from build123d import *

# Parameters (mm, degrees)
SKETCH1_R           = 2.1
BOSS_EXTRUDE1_DEPTH = 3
SKETCH2_W           = 4
SKETCH2_H           = 24
BOSS_EXTRUDE2_DEPTH = 15
SKETCH5_R           = 2.1
CUT_EXTRUDE3_DEPTH  = 65
FILLET2_R           = 2
FILLET3_R           = 3
SKETCH6_W           = 30
SKETCH6_H           = 5
BOSS_EXTRUDE3_DEPTH = 8
FILLET5_R           = 2
SKETCH9_R           = 2.1
CUT_EXTRUDE8_DEPTH  = 34


with BuildPart() as part:
    # Sketch1 → Boss-Extrude1 (new body)
    with BuildSketch(Plane(origin=(0, 0, 0), x_dir=(1, 0, 0), z_dir=(0, 1, 0))):
        Polygon((-20.9, -20.9), (20.9, -20.9), (20.9, -12), (28, -12), (28, 12), (20.9, 12), (20.9, 20.9), (-20.9, 20.9), (-20.9, 12), (-28, 12), (-28, -12), (-20.9, -12), align=None)
        with Locations(Location((-16, 16, 0), (0, 0, 270))):
            Circle(SKETCH1_R, mode=Mode.SUBTRACT)
        with Locations(Location((16, 16, 0), (0, 0, 270))):
            Circle(SKETCH1_R, mode=Mode.SUBTRACT)
        with Locations(Location((16, -16, 0), (0, 0, 270))):
            Circle(SKETCH1_R, mode=Mode.SUBTRACT)
        with Locations(Location((-16, -16, 0), (0, 0, 270))):
            Circle(SKETCH1_R, mode=Mode.SUBTRACT)
    extrude(amount=BOSS_EXTRUDE1_DEPTH)

    # Sketch2 → Boss-Extrude2 (add)
    with BuildSketch(Plane(origin=(0, 3, 0), x_dir=(1, 0, 0), z_dir=(0, 1, 0))):
        with Locations((-26, 0)):
            Rectangle(SKETCH2_W, SKETCH2_H)
        with Locations((26, 0)):
            Rectangle(SKETCH2_W, SKETCH2_H)
    extrude(amount=-BOSS_EXTRUDE2_DEPTH)

    # Sketch5 → Cut-Extrude3 (cut)
    with BuildSketch(Plane.ZY.offset(28)):
        with Locations((-7.999616758, -8)):
            Circle(SKETCH5_R)
        with Locations((7.999616758, -8)):
            Circle(SKETCH5_R)
    extrude(amount=-CUT_EXTRUDE3_DEPTH, mode=Mode.SUBTRACT)

    # Fillet2
    fillet2_edges = [part.edges().sort_by_distance(p)[0] for p in [
        (-20.9, 1.5, -12),
        (-20.9, 1.5, -20.9),
        (20.9, 1.5, -20.9),
        (20.9, 1.5, -12),
        (20.9, 1.5, 12),
        (20.9, 1.5, 20.9),
        (-20.9, 1.5, 20.9),
        (-20.9, 1.5, 12),
        (-26, -12, -12),
        (-26, -12, 12),
        (26, -12, 12),
        (26, -12, -12),
    ]]
    fillet(fillet2_edges, radius=FILLET2_R)

    # Fillet3
    fillet3_edges = [part.edges().sort_by_distance(p)[0] for p in [
        (28, 3, 0),
        (-28, 3, 0),
    ]]
    fillet(fillet3_edges, radius=FILLET3_R)

    # Sketch6 → Boss-Extrude3 (add)
    with BuildSketch(Plane(origin=(0, 3, 0), x_dir=(1, 0, 0), z_dir=(0, 1, 0))):
        with Locations((0, 7.992313958)):
            Rectangle(SKETCH6_W, SKETCH6_H)
        with Locations((0, -7.992313958)):
            Rectangle(SKETCH6_W, SKETCH6_H)
    extrude(amount=BOSS_EXTRUDE3_DEPTH)

    # Fillet5
    fillet5_edges = [part.edges().sort_by_distance(p)[0] for p in [
        (15, 3, 7.992313958),
        (-15, 3, 7.992313958),
        (15, 11, 7.992313958),
        (-15, 11, 7.992313958),
        (-15, 3, -7.992313958),
        (15, 3, -7.992313958),
        (-15, 11, -7.992313958),
        (15, 11, -7.992313958),
    ]]
    fillet(fillet5_edges, radius=FILLET5_R)

    # Sketch9 → Cut-Extrude8 (cut)
    with BuildSketch(Plane.XY.offset(10.492313958)):
        with Locations((-8, 7)):
            Circle(SKETCH9_R)
        with Locations((8, 7)):
            Circle(SKETCH9_R)
    extrude(amount=-CUT_EXTRUDE8_DEPTH, mode=Mode.SUBTRACT)


solid = part.part
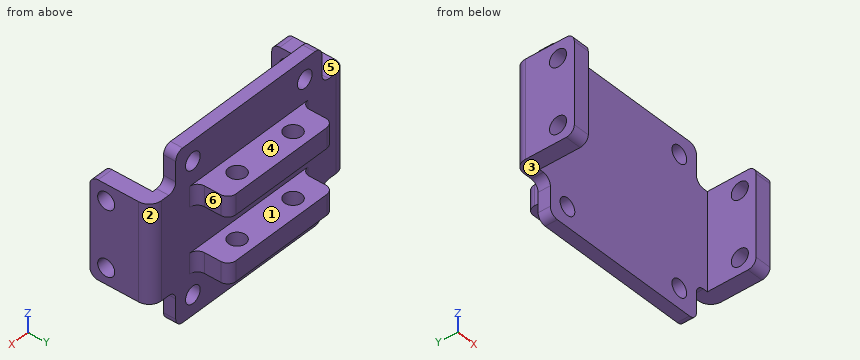
Could you check a few things on this model? Use its own coordinates, in mm. Face numbers are marked on the shaded views. A direction names the side the tool comes from. Give positions to 0.01 mm unless a question says otherwise; leave off trailing zeros. Write each loop counter-clockwise with the first axis right and the second up, starting at its lowest first coordinate (ties: lowest second). Pieces come first, ordered by that corner, then holes. Notation, with made-up numbers: (74.5, 77.25) -> (93.5, 77.25) arc R22 cw to (93.5, 101.25) -> close; hole circle Ø10 at (-36.5, 66). An arc over 180 degrees is marked (long way). Answer as a JSON object with one key per item and string values.
Q1. Suppose I cut it at D-D on y = -8. Write out the boundary of the cut face in (x, z).
Taken from the geometry:
{"outline": "(-28, -12) -> (-24, -12) -> (-24, -10.1) -> (-28, -10.1) -> close; (-28, -5.9) -> (-24, -5.9) -> (-24, 5.9) -> (-28, 5.9) -> close; (-28, 10.1) -> (-24, 10.1) -> (-24, 12) -> (-28, 12) -> close; (24, -12) -> (28, -12) -> (28, -10.1) -> (24, -10.1) -> close; (24, -5.9) -> (28, -5.9) -> (28, 5.9) -> (24, 5.9) -> close; (24, 10.1) -> (28, 10.1) -> (28, 12) -> (24, 12) -> close"}
Q2. Suppose I cut it at C-C on z = -16. Write out the boundary of the cut face in (x, y), then the cut area to 3 significant figures.
Taken from the geometry:
{"outline": "(-20.9, 0) -> (-18.1, 0) -> (-18.1, 3) -> (-20.9, 3) -> close; (-13.9, 0) -> (13.9, 0) -> (13.9, 3) -> (-13.9, 3) -> close; (18.1, 0) -> (20.9, 0) -> (20.9, 3) -> (18.1, 3) -> close", "area": "100 mm²"}
Q3. Suppose I cut it at A-A on y = -1.5. Write out the boundary of the cut face in (x, z).
Taken from the geometry:
{"outline": "(-28, -12) -> (-24, -12) -> (-24, 12) -> (-28, 12) -> close; (24, -12) -> (28, -12) -> (28, 12) -> (24, 12) -> close"}
Q4. We'd pull the mould along Z, two halves only. Please class the marked faces 1, 2 and 3: released by +Z, released by -Z, zero draft, split by the parting line, or undercut.
Taken from the geometry:
{"face 1": "undercut", "face 2": "zero draft", "face 3": "released by -Z"}
Q5. Please list where these lines run through material, in increasing order: L1, parallel to X at y = 0.8, z = 16; L2, parallel to Y at x = -8, z = 6; L3, parallel to X at y = -3.75, z = -1.5.
Taken from the geometry:
{"L1": "x = -20.9 to -18.1, -13.9 to 13.9, 18.1 to 20.9", "L2": "y = 0 to 4.9, 9.1 to 11", "L3": "x = -28 to -24, 24 to 28"}
Q6. Will these pins go through, and if not, where does the flat tip stop? pin 1 Ø1 at (x, z) = (3, -16.5) entering from -Y; pin 2 Ø5 at (x, y) = (8, 7) entering from +Z; pin 3 Ø2.5 at (x, y) = (-6, 6) entering from -Z.
Taken from the geometry:
{"pin 1": "stops at y = 0", "pin 2": "stops at z = 10.49", "pin 3": "stops at z = -10.49"}
Q7. Suppose I cut it at B-B on x = -8. Write out the boundary of the cut face in (y, z), then the cut area to 3 significant figures.
Taken from the geometry:
{"outline": "(0, -20.9) -> (3, -20.9) -> (3, -10.49) -> (4.9, -10.49) -> (4.9, -5.49) -> (3, -5.49) -> (3, 5.49) -> (4.9, 5.49) -> (4.9, 10.49) -> (3, 10.49) -> (3, 20.9) -> (0, 20.9) -> close; (9.1, -10.49) -> (11, -10.49) -> (11, -5.49) -> (9.1, -5.49) -> close; (9.1, 5.49) -> (11, 5.49) -> (11, 10.49) -> (9.1, 10.49) -> close", "area": "163 mm²"}
Q8. Which directions (+Z, -Z, +X, -X, +Y, -Y) give clear straight access to the entire face, cutting with the end or side of a thin tool? Please do the marked faces 4, 5 and 6.
Taken from the geometry:
{"face 4": "+Z, +X, -X, +Y", "face 5": "+Z, -X, +Y, -Y", "face 6": "+Z, -Z, +X, +Y"}
